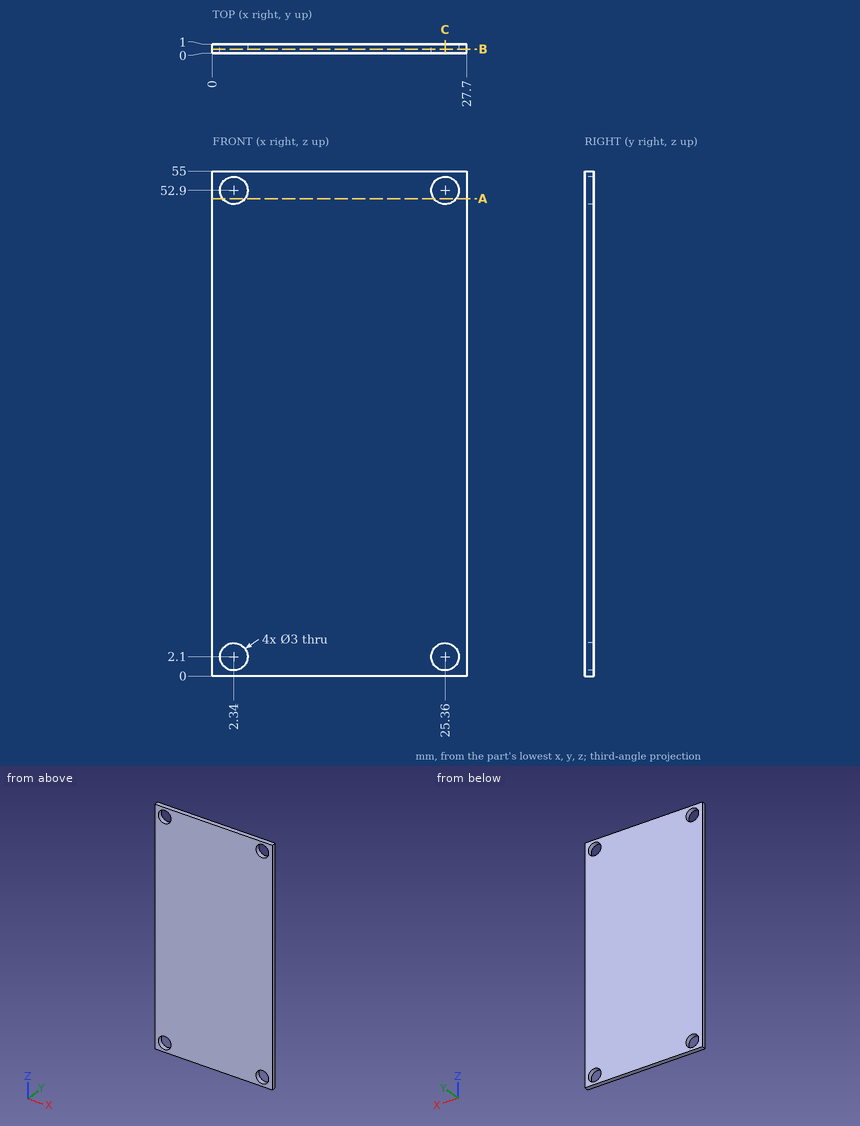
Can you work these out from the drawing? Everything is in mm from the part's minimum corner. Coordinates: 2 decimals unless noted, no trailing zeros. Loops run counter-clockwise (first coordinate to the right, second up) from the corner with the lowest first, then second, coordinate; pieces in that order, holes last. Notation, with made-up numbers: (34.25, -39.75) - (52.25, -39.75) arc R13 ccw to (52.25, -34.75) - close; hole circle Ø6 at (76.25, 88.25). An arc over 180 degrees is marked (long way). Put each result on its own line as item: value. Start each with the question number.
Item 1: If I drill on line 1 along Z through (x, y) = (2.34, 0.5); line 2 along Z through (x, y) = (26, 0.9); line 3 along X through (y, z) = (0.45, 3), over which ranges is the centre line in solid material (lowest first)?
Item 2: Suppose I cut it at A-A (z = 52). Please give me the cut outline in (x, y).
Item 3: Suppose I cut it at C-C (x = 25.36). Please give me the cut outline in (y, z), and give its area (3 significant figures).
Item 4: Suppose I cut it at B-B (y = 0.45). Please give me the cut outline in (x, z).
Item 5: For pin 1 (3.5 mm diameter, centred on x = 25.36, z = 52.9, fed in from +Y), with a flat end and sliding along its axis, tell me the tip position at first contact or that it passes through.
Here are the results:
1. line 1: 0 to 0.6, 3.6 to 51.4, 54.4 to 55
1. line 2: 0 to 0.74, 3.46 to 51.54, 54.26 to 55
1. line 3: 0 to 1.14, 3.54 to 24.16, 26.56 to 27.7
2. outline: (0, 0) - (1.14, 0) - (1.14, 1) - (0, 1) - close; (3.54, 0) - (24.16, 0) - (24.16, 1) - (3.54, 1) - close; (26.56, 0) - (27.7, 0) - (27.7, 1) - (26.56, 1) - close
3. outline: (0, 0) - (1, 0) - (1, 0.6) - (0, 0.6) - close; (0, 3.6) - (1, 3.6) - (1, 51.4) - (0, 51.4) - close; (0, 54.4) - (1, 54.4) - (1, 55) - (0, 55) - close
3. area: 49.0 mm²
4. outline: (0, 0) - (27.7, 0) - (27.7, 55) - (0, 55) - close; hole circle Ø3 at (2.34, 2.1); hole circle Ø3 at (2.34, 52.9); hole circle Ø3 at (25.36, 2.1); hole circle Ø3 at (25.36, 52.9)
5. pin 1: y = 1
